Autodesk Inventor part; units mm, degrees
ref_plane "YZ Plane" through (0, 0, 0) normal (1, 0, 0) x (0, 1, 0)
ref_plane "XZ Plane" through (0, 0, 0) normal (0, 1, 0) x (-1, 0, 0)
ref_plane "XY Plane" through (0, 0, 0) normal (0, 0, 1) x (1, 0, 0)
sketch "Sketch8" plane through (0, 0, 0) normal (0, 0, 1) x (1, 0, 0)
  circle A0 centre (0, 0) radius 39.5
  circle A1 centre (0, 0) radius 27
  line L0 (-23.6881, -23.6881) -> (23.6881, -23.6881) construction
  line L1 (23.6881, -23.6881) -> (23.6881, 23.6881) construction
  line L2 (23.6881, 23.6881) -> (-23.6881, 23.6881) construction
  line L3 (-23.6881, 23.6881) -> (-23.6881, -23.6881) construction
  line L4 (-23.6881, -23.6881) -> (23.6881, 23.6881) construction
  line L5 (23.6881, -23.6881) -> (-23.6881, 23.6881) construction
  circle A2 centre (-23.6881, 23.6881) radius 1.75
  circle A3 centre (23.6881, 23.6881) radius 1.75
  circle A4 centre (-23.6881, -23.6881) radius 1.75
  circle A5 centre (23.6881, -23.6881) radius 1.75
  dimension "d23" = 79
  dimension "d24" = 54
  dimension "d25" = 67
  dimension "d26" = 3.5
  dimension "d27" = 3.5
  dimension "d28" = 3.5
  dimension "d29" = 3.5
extrude "Extrusion8" add sketch "Sketch8" along normal blind 6
equation "\"d27\" = d26"
equation "\"d28\" = d26"
equation "\"d29\" = d26"
properties part number "2209B_Tube Flange Inner_V1" material "ABS Plastic"
Build history of the part. All positions in model axes, mm. Round coordinates to 2 decimals unless told otherwise and drop trailing zeros. Write each loop counter-clockwise with the first axis right and the second up, starting at its lowest first coordinate (ties: lowest second). Pieces come first, ordered by that corner, then holes. Notation, with made-up numbers: (-4.5, 54) - (42.5, 54) arc R34 cw to (42.5, 87) - close; hole circle Ø9 at (-38, -6). An arc over 180 degrees is marked (long way). Use CSV: the item, a comma, the result in double quotes.
(1) Band-saw the part on D-D (x = 34.5). Write the cut outline in (y, z).
Response:
outline,"(-19.24, 0) - (19.24, 0) - (19.24, 6) - (-19.24, 6) - close"
(2) Mould opens along Y. For faces 1 (the flat face through (8, -26, 6)), 2 (the cylindrical face through (-29.11, -26.7, 2.96)), 3 (the cylindrical face through (-5.85, 26.36, 2.96)) say: pulls with the +Y half, pulls with the -Y half, needs draft (parallel to the pull), parting line crosses it, or undercut.
Response:
face 1,"needs draft"
face 2,"parting line crosses it"
face 3,"undercut"
(3) Wall check: line 1 (Y direction, x = 0, z = 3.25); line 2 (X direction, y = -25, z = 1.35); line 3 (Y direction, x = -24.5, z = 1.2). Give the ranges that are in metal, low to high.
Response:
line 1,"-39.5 to -27, 27 to 39.5"
line 2,"-30.58 to -24.85, -22.53 to -10.2, 10.2 to 22.53, 24.85 to 30.58"
line 3,"-30.98 to -25.24, -22.14 to -11.35, 11.35 to 22.14, 25.24 to 30.98"
(4) Band-saw the part on A-A (y = 0). Write the cut outline in (x, z).
Response:
outline,"(-39.5, 0) - (-27, 0) - (-27, 6) - (-39.5, 6) - close; (27, 0) - (39.5, 0) - (39.5, 6) - (27, 6) - close"
(5) Band-saw the part on C-C (z = 4.3). Write the cut outline in (x, y), plus the area to 3 significant figures.
Response:
outline,"circle Ø79 at (0, 0); hole circle Ø54 at (0, 0); hole circle Ø3.5 at (-23.69, -23.69); hole circle Ø3.5 at (-23.69, 23.69); hole circle Ø3.5 at (23.69, -23.69); hole circle Ø3.5 at (23.69, 23.69)"
area,"2,570 mm²"
(6) Pin check, flat tip, straight feed: P1, Ø1.5, axis at y = -7.5, z = 4.5, coming from the -X side. Stop position of the tip, or through.
Response:
P1,"x = -38.92"
